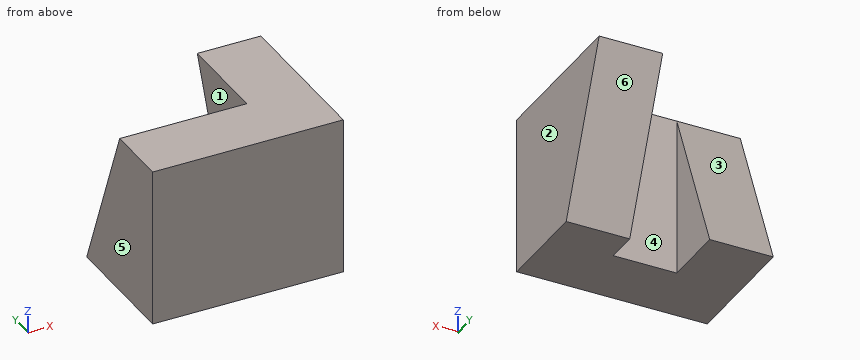
from build123d import *

# Parameters (mm, degrees)
BOSS_EXTRUDE1_DEPTH = 25
BOSS_EXTRUDE2_DEPTH = 10
BOSS_EXTRUDE3_DEPTH = 10


with BuildPart() as part:
    # Sketch1 → Boss-Extrude1 (new body)
    with BuildSketch(Plane.XY):
        Polygon((-30, 10), (-10, 10), (-10, 15), (0, 15), (0, 0), (-30, 0), align=None)
    extrude(amount=BOSS_EXTRUDE1_DEPTH)

    # Sketch2 → Boss-Extrude2 (add)
    with BuildSketch(Plane.ZY.offset(30)):
        Polygon((0, 10), (0, 20), (25, 10), align=None)
    extrude(amount=-BOSS_EXTRUDE2_DEPTH)

    # Sketch3 → Boss-Extrude3 (add)
    with BuildSketch(Plane(origin=(0, 0, 0), x_dir=(0, 0, -1), z_dir=(1, 0, 0))):
        Polygon((-25, 15), (-25, 25), (0, 15), align=None)
    extrude(amount=-BOSS_EXTRUDE3_DEPTH)


solid = part.part
Input: part model. Units: mm. Frame: model coordinates. Face numbers are marked on the shaded views. A direction names the side the tool comes from. Give positions to 0.01 mm unless a question says otherwise; leave off trailing zeros. Write each loop counter-clockwise with the first axis right and the second up, starting at its lowest first coordinate (ties: lowest second). Pieces come first, ordered by that corner, then holes.
Q1. Set-up query: the marked faces 1, 2 and 3. Return all of +Z, -Z, +X, -X, +Y, -Y with unobstructed straight access to the full face (end or side cutting, diameter ignored); none if empty.
Q2. Material intervals for probe 1 along X at (y, z) = (13.75, 11); probe 2 along Y at (x, z) = (-19.5, 21.5); probe 3 along X at (y, z) = (17.5, 2.25), sorted ascending.
Q3. Pull-direction query (X, two-part tool) for the marked faces 4, 5 and 6; classes: pulls with the +X half, pulls with the -X half, needs draft (parallel to the pull), parting line crosses it, or undercut.
Q4. Section A-A, the plane y = 11. Output: boundary loops of the cut face in (x, z).
Q5. First-contact query: P1, Ø1, axis at y = 19.5, z = 15, coming from the -X side; P2, Ø5, axis at x = -15, z = 17.5, coming from the +Y side; P3, Ø1, axis at x = -6.5, z = 4, coming from the +Y side. Flat tips, straight axial feed; report the tip coordinate or a pass-through.
Q6. Section B-B, the plane y = 13.5. Output: boundary loops of the cut face in (x, z), plus the area to 4 significant figures.
Q7. Section C-C, the plane z = 14.75. Output: boundary loops of the cut face in (x, y).
Q8. Section D-D, the plane x = -27. Output: boundary loops of the cut face in (y, z), plus the area to 3 significant figures.
Filled in:
1. face 1: +Z, -Z, +Y
1. face 2: +Z, -Z, +X, +Y, -Y
1. face 3: +Z, -X, +Y
2. probe 1: x = -30 to -20, -10 to 0
2. probe 2: y = 0 to 10
2. probe 3: x = -30 to -20
3. face 4: undercut
3. face 5: pulls with the -X half
3. face 6: needs draft
4. outline: (-30, 0) - (-20, 0) - (-20, 22.5) - (-30, 22.5) - close; (-10, 0) - (0, 0) - (0, 25) - (-10, 25) - close
5. P1: stops at x = -10
5. P2: stops at y = 10
5. P3: stops at y = 16.8
6. outline: (-30, 0) - (-20, 0) - (-20, 16.25) - (-30, 16.25) - close; (-10, 0) - (0, 0) - (0, 25) - (-10, 25) - close
6. area: 412.5 mm2
7. outline: (-30, 0) - (0, 0) - (0, 20.9) - (-10, 20.9) - (-10, 10) - (-20, 10) - (-20, 14.1) - (-30, 14.1) - close
8. outline: (0, 0) - (20, 0) - (10, 25) - (0, 25) - close
8. area: 375 mm2
